Geometry check sheet. Reference: the model listing, model coordinates, mm. A direction names the side the tool comes from. Round coordinates to 2 decimals unless told otherwise and drop trailing zeros. Order: outer loops, then holes, each group sorted by start corner. A loop starts at its lowest first (then second) coordinate and runs counter-clockwise, first axis right, second up. Notation, with made-up numbers: (19, -3) - (26, -3) arc R11 ccw to (26, 9) - close; hole circle Ø2 at (9, 87). An arc over 180 degrees is marked (long way). Use a Markdown table: item, result. Add a question column.
(1) Thickness scan on line 1 along X through (y, z) = (-14, 2.85); line 2 along Y through (x, z) = (0, 2.1); line 3 along Y through (x, z) = (-0.5, 3.4). Record the ranges inside material, lowest first. Write a range as [from, to].
(2) Section check C-C on z = 2.55. Record the boundary of the cut face in (x, y), then the cut area to 3 significant figures.
(3) Section check B-B on x = 0. Record the boundary of the cut face in (y, z).
(4) Section check A-A on y = -5. Record the boundary of the cut face in (x, z).
(5) Section check D-D on y = -18.5. Record the boundary of the cut face in (x, z), then the cut area to 3 significant figures.
(6) Mould release check, pull along X, two halves, no side actions. Record for faces 1 (the face through (15.405, 0, 3)), 2 (the face through (0, 0, 0)), 3 (the face through (22.5, 0, 3)), 4 (the face through (-7.987, 0, 3)): released by +X, released by -X, zero draft, split by the parting line, or undercut.
(7) Gauge pin test, flat end, axial feed: P1, Ø4.5, axis at x = 0, y = -18.5, coming from the -Z side. Record the tip position at first contact, or that the pin passes through.
(8) Access from +Z, -Z, +X, -X, +Y, -Y to the whole of each face (thin tool, end or side, straight path). Record for faces 5 (the face through (0, -30, 3)), 6 (the face through (-11.63, 20.263, 2.958)).
```python
from build123d import *

# Parameters (mm, degrees)
SKETCH1_W           = 45
SKETCH1_H           = 60
SKETCH1_R           = 2.5
BOSS_EXTRUDE1_DEPTH = 6


with BuildPart() as part:
    # Sketch1 → Boss-Extrude1 (new body)
    with BuildSketch(Plane(origin=(0, 0, 0), x_dir=(-1, 0, 0), z_dir=(0, 0, -1))):
        Rectangle(SKETCH1_W, SKETCH1_H)
        with Locations((0, 18.5)):
            Circle(SKETCH1_R, mode=Mode.SUBTRACT)
        with Locations((0, -18.5)):
            Circle(SKETCH1_R, mode=Mode.SUBTRACT)
        with BuildLine():
            Line((-8.277280201, 16.7), (-8.277280201, -16.7))
            ThreePointArc((-8.277280201, -16.7), (-11.841231537, -20.263951335), (-15.405182872, -16.7))
            Line((-15.405182872, -16.7), (-15.405182872, 16.7))
            ThreePointArc((-15.405182872, 16.7), (-11.841231537, 20.263951335), (-8.277280201, 16.7))
        make_face(mode=Mode.SUBTRACT)
        with BuildLine():
            Line((7.987422003, 16.7), (7.987422003, -16.7))
            ThreePointArc((7.987422003, -16.7), (11.551373339, -20.263951335), (15.115324674, -16.7))
            Line((15.115324674, -16.7), (15.115324674, 16.7))
            ThreePointArc((15.115324674, 16.7), (11.551373339, 20.263951335), (7.987422003, 16.7))
        make_face(mode=Mode.SUBTRACT)
    extrude(amount=-BOSS_EXTRUDE1_DEPTH)


solid = part.part
```
Check sheet entries:
| question | item | result |
|---|---|---|
| 1 | line 1 | x = [-22.5, -15.12], [-7.99, 8.28], [15.41, 22.5] |
| 1 | line 2 | y = [-30, -21], [-16, 16], [21, 30] |
| 1 | line 3 | y = [-30, -20.95], [-16.05, 16.05], [20.95, 30] |
| 2 | outline | (-22.5, -30) - (22.5, -30) - (22.5, 30) - (-22.5, 30) - close; hole (-15.12, -16.7) arc R3.56 ccw to (-7.99, -16.7) - (-7.99, 16.7) arc R3.56 ccw to (-15.12, 16.7) - close; hole circle Ø5 at (0, -18.5); hole circle Ø5 at (0, 18.5); hole (8.28, -16.7) arc R3.56 ccw to (15.41, -16.7) - (15.41, 16.7) arc R3.56 ccw to (8.28, 16.7) - close |
| 2 | area | 2,100 mm2 |
| 3 | outline | (-30, 0) - (-21, 0) - (-21, 6) - (-30, 6) - close; (-16, 0) - (16, 0) - (16, 6) - (-16, 6) - close; (21, 0) - (30, 0) - (30, 6) - (21, 6) - close |
| 4 | outline | (-22.5, 0) - (-15.12, 0) - (-15.12, 6) - (-22.5, 6) - close; (-7.99, 0) - (8.28, 0) - (8.28, 6) - (-7.99, 6) - close; (15.41, 0) - (22.5, 0) - (22.5, 6) - (15.41, 6) - close |
| 5 | outline | (-22.5, 0) - (-14.63, 0) - (-14.63, 6) - (-22.5, 6) - close; (-8.48, 0) - (-2.5, 0) - (-2.5, 6) - (-8.48, 6) - close; (2.5, 0) - (8.77, 0) - (8.77, 6) - (2.5, 6) - close; (14.92, 0) - (22.5, 0) - (22.5, 6) - (14.92, 6) - close |
| 5 | area | 166 mm2 |
| 6 | face 1 | undercut |
| 6 | face 2 | zero draft |
| 6 | face 3 | released by +X |
| 6 | face 4 | undercut |
| 7 | P1 | passes through |
| 8 | face 5 | +Z, -Z, +X, -X, -Y |
| 8 | face 6 | +Z, -Z |
